The listing builds one solid part. Answer for the finished solid, in the listing's coordinates (mm). Face numbers are marked on the shaded views. A direction names the side the tool comes from. Give positions to 0.01 mm unless a question says otherwise; leave off trailing zeros. Order: outer loops, then holes, each group sorted by start corner. A loop starts at its lowest first (then second) coordinate and runs counter-clockwise, first axis right, second up. Notation, with made-up numbers: (-18.75, -13) - (10.25, -13) arc R27 cw to (10.25, 20) - close; hole circle Ø8 at (17, 52.25). An arc over 180 degrees is marked (long way). Answer in a Markdown table with one row per item.
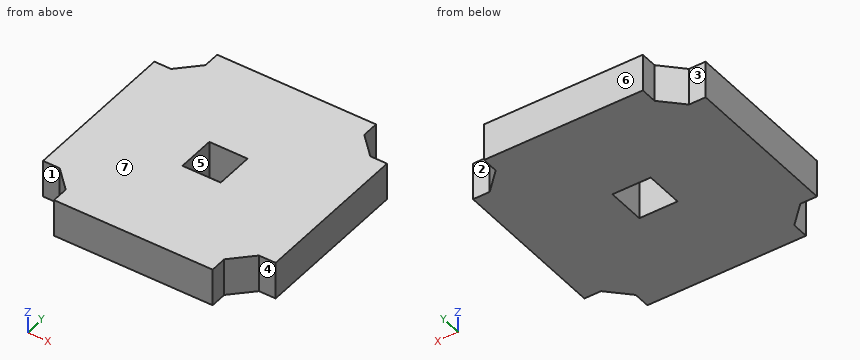
Autodesk Inventor part; units mm, degrees
ref_plane "Work Plane1" through (0, 0, 10) normal (0, 0, 1) x (1, 0, 0)
ref_plane "YZ Plane" through (0, 0, 0) normal (1, 0, 0) x (0, 1, 0)
ref_plane "XZ Plane" through (0, 0, 0) normal (0, 1, 0) x (-1, 0, 0)
ref_plane "Work Plane1" through (0, 0, 10) normal (0, 0, 1) x (1, 0, 0)
sketch "Sketch1" plane through (0, 0, 10) normal (0, 0, 1) x (1, 0, 0)
  line L0 (-4.0299, -0.3538) -> (-2.2322, 1.4439) construction
  arc A0 (-1.4439, 2.2322) -> (-2.2322, 1.4439) centre (-0.9299, 0.9299) ccw construction
  line L1 (-1.4439, 2.2322) -> (0.3538, 4.0299) construction
  line L2 (-37.8299, 42.8299) -> (-37.8299, 37.8299) construction
  line L3 (-37.8299, 37.8299) -> (-42.9208, 37.8299) construction
  line L4 (-37.8299, 42.2137) -> (-37.8299, 45.8299) construction
  line L5 (-37.8299, 45.8299) -> (-4.0299, 45.8299) construction
  line L6 (-4.0299, 45.8299) -> (-4.0299, 42.2137) construction
  line L7 (-4.0299, 4.0299) -> (0.3538, 4.0299)
  circle A1 centre (-20.9299, 20.9299) radius 17.5
  line L8 (-20.9299, 58.9723) -> (17.1124, 20.9299) construction
  line L9 (17.1124, 20.9299) -> (-20.9299, -17.1124) construction
  line L10 (-20.9299, -17.1124) -> (-58.9723, 20.9299) construction
  line L11 (-58.9723, 20.9299) -> (-20.9299, 58.9723) construction
  line L12 (-20.9299, 58.9723) -> (-20.9299, -17.1124) construction
  line L13 (17.1124, 20.9299) -> (-58.9723, 20.9299) construction
  line L14 (-20.9299, 58.9723) -> (32.8701, 58.9723) construction
  line L15 (-43.4299, 43.4299) -> (1.5701, 43.4299) construction
  line L16 (1.5701, 43.4299) -> (1.5701, -1.5701) construction
  line L17 (1.5701, -1.5701) -> (-43.4299, -1.5701) construction
  line L18 (-43.4299, -1.5701) -> (-43.4299, 43.4299) construction
  line L19 (-43.4299, 43.4299) -> (1.5701, -1.5701) construction
  line L20 (1.5701, 43.4299) -> (-43.4299, -1.5701) construction
  line L21 (-43.4299, 5.3876) -> (-43.4299, 36.4723)
  line L22 (-43.4299, 36.4723) -> (-36.4723, 43.4299)
  line L23 (-36.4723, 43.4299) -> (-5.3876, 43.4299)
  line L24 (-5.3876, 43.4299) -> (1.5701, 36.4723)
  line L25 (1.5701, 36.4723) -> (1.5701, 5.3876)
  line L26 (1.5701, 5.3876) -> (-5.3876, -1.5701)
  line L27 (-5.3876, -1.5701) -> (-36.4723, -1.5701)
  line L28 (-36.4723, -1.5701) -> (-43.4299, 5.3876)
  line L29 (-4.0299, 42.2137) -> (-37.8299, 42.2137)
  line L30 (-4.0299, -0.3538) -> (-4.0299, 4.0299)
  circle A2 centre (-20.9299, 20.9299) radius 1.5
  line L31 (-10.9299, 10.9299) -> (-30.9299, 10.9299) construction
  line L32 (-30.9299, 10.9299) -> (-30.9299, 30.9299) construction
  line L33 (-30.9299, 30.9299) -> (-10.9299, 30.9299) construction
  line L34 (-10.9299, 30.9299) -> (-10.9299, 10.9299) construction
  line L35 (-10.9299, 10.9299) -> (-30.9299, 30.9299) construction
  line L36 (-30.9299, 10.9299) -> (-10.9299, 30.9299) construction
  circle A3 centre (-30.9299, 30.9299) radius 1.4
  circle A4 centre (-30.9299, 10.9299) radius 1.4
  circle A5 centre (-10.9299, 10.9299) radius 1.4
  line L37 (-45.8299, 37.8299) -> (-42.0723, 37.8299) construction
  line L38 (-42.1723, 37.7299) -> (-45.8299, 37.7299)
  line L39 (-45.8299, 37.7299) -> (-45.8299, 4.1299)
  line L40 (-45.8299, 4.1299) -> (-42.1723, 4.1299)
  line L41 (-42.1723, 4.1299) -> (-42.1723, 37.7299)
  line L42 (-45.8299, 4.0299) -> (-42.0723, 4.0299) construction
  line L43 (-45.8299, 37.8299) -> (-42.0723, 37.8299)
  line L44 (-37.7299, 45.8299) -> (-4.1299, 45.8299)
  line L45 (-4.1299, 45.8299) -> (-4.1299, 42.1723)
  line L46 (-4.1299, 42.1723) -> (-37.7299, 42.1723)
  line L47 (-37.7299, 42.1723) -> (-37.7299, 45.8299)
  line L48 (0.4701, 37.8299) -> (0.4701, 4.0299) construction
  line L49 (0.4701, 4.0299) -> (3.9701, 4.0299) construction
  line L50 (3.9701, 37.8299) -> (3.9701, 4.0299) construction
  line L51 (0.4701, 37.8299) -> (3.9701, 37.8299) construction
  line L52 (-45.8299, -3.9701) -> (-4.0299, -3.9701) construction
  line L53 (0.3124, 37.7299) -> (3.9701, 37.7299)
  line L54 (3.9701, 37.7299) -> (3.9701, 4.1299)
  line L55 (3.9701, 4.1299) -> (0.3124, 4.1299)
  line L56 (0.3124, 4.1299) -> (0.3124, 37.7299)
  line L57 (-4.1713, -0.3538) -> (-37.7299, -0.3538)
  line L58 (-37.7299, -0.3538) -> (-37.7299, -3.9701)
  line L59 (-37.7299, -3.9701) -> (-4.1713, -3.9701)
  line L60 (-4.1713, -3.9701) -> (-4.1713, -0.3538)
  point P0 (-37.8299, 4.0299)
  dimension "d18" = 53.8
  dimension "d19" = 45
  dimension "d20" = 53.8
  dimension "d21" = 45
  dimension "d22" = 45
  dimension "d30" = 20
  dimension "d31" = 20
  dimension "d32" = 2.8
  dimension "d33" = 2.8
  dimension "d34" = 2.8
  dimension "d35" = 3
  dimension "d36" = 0.1
  dimension "d37" = 0.1
  dimension "d38" = 0.1
  dimension "d39" = 0.1
extrude "Extrusion1" add sketch "Sketch1" along normal blind 8 contours L30 L26 L57 L28 L41 L22 L46 L24 L56 L7 | L7 L26 L30 | L56 L24 L25 L26 | L26 L25 L24 L53 L54 L55 | L60 L59 L58 L57 L28 L27 L26 | L26 L27 L28 L57 | L46 L22 L29 L24 | L24 L29 L45 | L40 L39 L38 L22 L21 L28 | L28 L21 L22 L41 | L29 L22 L23 L24 | L24 L23 L22 L29 L47 L44 L45 | L47 L29 L22 | A1 | A2 | A3 | A4 | A5
sketch "Skizze4" plane through (0, 0, 18) normal (0, 0, 1) x (1, 0, 0)
  line L0 (-37.7299, 42.1723) -> (-42.1723, 37.7299)
  line L1 (-42.1723, 37.7299) -> (-45.8299, 37.7299)
  line L2 (-45.8299, 37.7299) -> (-45.8299, 4.1299) construction
  line L3 (-45.8299, 4.1299) -> (-42.1723, 4.1299)
  line L4 (-42.1723, 4.1299) -> (-37.6885, -0.3538)
  line L5 (-37.6885, -0.3538) -> (-37.7299, -0.3538)
  line L6 (-37.7299, -0.3538) -> (-37.7299, -3.9701)
  line L7 (-37.7299, -3.9701) -> (-4.1713, -3.9701) construction
  line L8 (-4.1713, -3.9701) -> (-4.1713, -0.3538)
  line L9 (-4.1713, -0.3538) -> (0.3124, 4.1299)
  line L10 (0.3124, 4.1299) -> (3.9701, 4.1299)
  line L11 (3.9701, 4.1299) -> (3.9701, 37.7299) construction
  line L12 (3.9701, 37.7299) -> (0.3124, 37.7299)
  line L13 (0.3124, 37.7299) -> (-4.1299, 42.1723)
  line L14 (-4.1299, 42.1723) -> (-4.1299, 45.8299)
  line L15 (-4.1299, 45.8299) -> (-37.7299, 45.8299) construction
  line L16 (-37.7299, 45.8299) -> (-37.7299, 42.1723)
  line L17 (-37.9299, 46.0299) -> (-3.9299, 46.0299) construction
  line L18 (-3.9299, 46.0299) -> (-3.9299, 42.2551)
  line L19 (-3.9299, 42.2551) -> (0.3953, 37.9299)
  line L20 (0.3953, 37.9299) -> (4.1701, 37.9299)
  line L21 (4.1701, 37.9299) -> (4.1701, 3.9299) construction
  line L22 (4.1701, 3.9299) -> (0.3953, 3.9299)
  line L23 (0.3953, 3.9299) -> (-3.9713, -0.4367)
  line L24 (-3.9713, -0.4367) -> (-3.9713, -4.1701)
  line L25 (-3.9713, -4.1701) -> (-37.9299, -4.1701) construction
  line L26 (-37.9299, -4.1701) -> (-37.9299, -0.3953)
  line L27 (-37.9299, -0.3953) -> (-42.2551, 3.9299)
  line L28 (-42.2551, 3.9299) -> (-46.0299, 3.9299)
  line L29 (-46.0299, 3.9299) -> (-46.0299, 37.9299) construction
  line L30 (-46.0299, 37.9299) -> (-42.2551, 37.9299)
  line L31 (-42.2551, 37.9299) -> (-37.9299, 42.2551)
  line L32 (-37.9299, 42.2551) -> (-37.9299, 46.0299)
  line L33 (-45.8299, 37.7299) -> (-45.8299, 37.9299)
  line L34 (-4.1299, 45.8299) -> (-37.7299, 45.8299)
  line L35 (-37.7299, 45.8299) -> (-37.9299, 45.8299)
  line L36 (-4.1299, 45.8299) -> (-3.9299, 45.8299)
  line L37 (3.9701, 37.7299) -> (3.9701, 37.9299)
  line L38 (3.9701, 4.1299) -> (3.9701, 37.7299)
  line L39 (3.9701, 4.1299) -> (3.9701, 3.9299)
  line L40 (-4.1713, -3.9701) -> (-3.9713, -3.9701)
  line L41 (-37.7299, -3.9701) -> (-37.9299, -3.9701)
  line L42 (-45.8299, 4.1299) -> (-45.8299, 3.9299)
  point P0 (0, 0)
  dimension "d40" = 0.2
extrude "IM_offset" add sketch "Skizze4" against normal up to surface (8 mm away)
ref_plane "Arbeitsebene5" through (-37.9299, 20.9299, 10) normal (0, -1, 0) x (1, 0, 0)
ref_plane "Arbeitsebene6" through (-20.9299, 3.9299, 10) normal (-1, 0, 0) x (0, 0, 1)
sketch "Skizze27" plane through (-37.9299, 20.9299, 10) normal (0, -1, 0) x (1, 0, 0)
  line L0 (17, -13.6) -> (17, 11.6)
  point P0 (37.9299, -10)
sketch "Skizze31" plane through (0, 0, 18) normal (0, 0, 1) x (1, 0, 0)
  line L0 (-3.9299, 45.8299) -> (-37.9299, 45.8299)
  line L1 (-37.9299, 45.8299) -> (-37.9299, 42.2551)
  line L2 (-37.9299, 42.2551) -> (-42.2551, 37.9299)
  line L3 (-42.2551, 37.9299) -> (-45.8299, 37.9299)
  line L4 (-45.8299, 37.9299) -> (-45.8299, 3.9299)
  line L5 (-42.2551, 3.9299) -> (-45.8299, 3.9299)
  line L6 (-37.9299, -0.3953) -> (-42.2551, 3.9299)
  line L7 (-37.9299, -3.9701) -> (-37.9299, -0.3953)
  line L8 (-3.9713, -3.9701) -> (-37.9299, -3.9701)
  line L9 (-3.9713, -3.9701) -> (-3.9713, -0.4367)
  line L10 (-3.9713, -0.4367) -> (0.3953, 3.9299)
  line L11 (0.3953, 3.9299) -> (3.9701, 3.9299)
  line L12 (3.9701, 3.9299) -> (3.9701, 37.9299)
  line L13 (3.9701, 37.9299) -> (0.3953, 37.9299)
  line L14 (0.3953, 37.9299) -> (-3.9299, 42.2551)
  line L15 (-3.9299, 42.2551) -> (-3.9299, 45.8299)
  line L16 (-3.9713, -3.9701) -> (-37.9299, -3.9701)
  line L17 (-45.9799, 54.3054) -> (-45.9799, 21.9906)
  line L18 (-3.9299, 45.8299) -> (-37.9299, 45.8299)
  circle A0 centre (-20.9299, 20.9299) radius 24.9 construction
  line L19 (-25.0299, 25.0299) -> (-16.8299, 25.0299)
  line L20 (-16.8299, 25.0299) -> (-16.8299, 16.8299)
  line L21 (-16.8299, 16.8299) -> (-25.0299, 16.8299)
  line L22 (-25.0299, 16.8299) -> (-25.0299, 25.0299)
  line L23 (-25.0299, 25.0299) -> (-16.8299, 16.8299)
  line L24 (-16.8299, 25.0299) -> (-25.0299, 16.8299)
  point P0 (0, 0)
  dimension "d169" = 8.2
  dimension "d170" = 8.2
extrude "Extrusion26" cut sketch "Skizze31" against normal blind 10 contours L23 L24 L22 | L19 L24 L23 | L20 L23 L24 | L24 L23 L21
properties part number "20_Cube_Insert_ESP32Cam_angle_v3"
Item 1: Which of the six approach directions +Z, -Z, +X, -X, +Y, -Y give full straight-line access (tool end or side, diameter ignored) to the marked faces 1, 2, 3 and 4?
Answer block:
| item | result |
|---|---|
| face 1 | +Z, -Z, -X, -Y |
| face 2 | +Z, -Z, +X, +Y |
| face 3 | +Z, -Z, -X, +Y |
| face 4 | +Z, -Z, +X, -Y |
Item 2: Find section C-C on x = -43. Write down the section's boundary in (y, z), then the cut area to 3 significant figures.
Answer block:
| item | result |
|---|---|
| outline | (3.93, 10) - (37.93, 10) - (37.93, 18) - (3.93, 18) - close |
| area | 272 mm² |
Item 3: Find section D-D on y = 2. Write down the section's boundary in (x, z), then the cut area to 3 significant figures.
Answer block:
| item | result |
|---|---|
| outline | (-40.33, 10) - (-1.53, 10) - (-1.53, 18) - (-40.33, 18) - close |
| area | 310 mm² |
Item 4: Find section B-B on z = 11. Write down the section's boundary in (x, y).
Answer block:
| item | result |
|---|---|
| outline | (-45.83, 3.93) - (-42.26, 3.93) - (-37.93, -0.4) - (-37.93, -3.97) - (-3.97, -3.97) - (-3.97, -0.44) - (0.4, 3.93) - (3.97, 3.93) - (3.97, 37.93) - (0.4, 37.93) - (-3.93, 42.26) - (-3.93, 45.83) - (-37.93, 45.83) - (-37.93, 42.26) - (-42.26, 37.93) - (-45.83, 37.93) - close; hole (-25.03, 16.83) - (-16.83, 16.83) - (-16.83, 25.03) - (-25.03, 25.03) - close |
Item 5: Find section A-A on y = 21.5. Write down the section's boundary in (x, z), then the cut area to 3 significant figures.
Answer block:
| item | result |
|---|---|
| outline | (-45.83, 10) - (-25.03, 10) - (-25.03, 18) - (-45.83, 18) - close; (-16.83, 10) - (3.97, 10) - (3.97, 18) - (-16.83, 18) - close |
| area | 333 mm² |
Item 6: Consider line 1 (Y direction, x = -19, z = 17); line 2 (X direction, y = 18, z = 12.75); line 3 (X direction, y = 43, z = 13). Determine where each line is inside the solid, lowest interval first.
Answer block:
| item | result |
|---|---|
| line 1 | -3.97 to 16.83, 25.03 to 45.83 |
| line 2 | -45.83 to -25.03, -16.83 to 3.97 |
| line 3 | -37.93 to -3.93 |
Item 7: Each of these flat-tipped pins is pushed along its axis until it touches: P1, Ø4, axis at y = -2, z = 14, coming from the +X side; P2, Ø4, axis at x = 3, z = 12, coming from the -Y side; P3, Ø3, axis at y = 2, z = 16.5, coming from the -X side. Where does it stop, or does it pass through?
Answer block:
| item | result |
|---|---|
| P1 | x = -3.53 |
| P2 | y = 3.93 |
| P3 | x = -41.83 |
Item 8: Determine the mould class of the marked faces 5, 6 and 7 for opening direction Y: pulls with the +Y half, pulls with the -Y half, needs draft (parallel to the pull), parting line crosses it, or undercut.
Answer block:
| item | result |
|---|---|
| face 5 | undercut |
| face 6 | pulls with the +Y half |
| face 7 | needs draft |
